Read the model definition and answer for the solid it produces. Units are mm, in the model's axes. Face numbers are marked on the shaded views. Round coordinates to 2 decimals unless told otherwise and drop trailing zeros. Write each loop counter-clockwise with the first axis right and the second up, starting at its lowest first coordinate (ties: lowest second). Pieces come first, ordered by that corner, then holes.
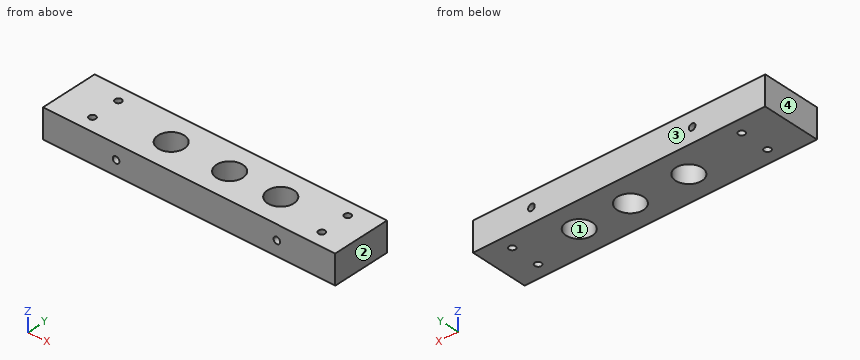
from build123d import *

# Parameters (mm, degrees)
F_200X40X20_START          = -10
SKETCH_1_W                 = 200
SKETCH_1_H                 = 40
F_200X40X20_DEPTH          = 20
CUT_EXTRUDE_321_DEPTH      = 202.246117975
CUT_EXTRUDE_321_DEPTH_BACK = 202.246117975
SKETCH_2_R                 = 9
SKETCH_2_R_2               = 2.25
CUT_EXTRUDE_M4_DEPTH       = 202.246117975
CUT_EXTRUDE_M4_DEPTH_BACK  = 202.246117975
SKETCH_3_R                 = 2.25


with BuildPart() as part:
    # 草图1 → 前臂200x40x20 (new body)
    with BuildSketch(Plane.XY.offset(F_200X40X20_START)):
        with Locations((100, 0)):
            Rectangle(SKETCH_1_W, SKETCH_1_H)
    extrude(amount=F_200X40X20_DEPTH)

    # 草图2 → Cut-Extrude 321 (cut, two sides: drawn at the far end of the back side and taken through both)
    with BuildSketch(Plane.XY.offset(-CUT_EXTRUDE_321_DEPTH_BACK)):
        with Locations((70, 0)):
            Circle(SKETCH_2_R)
        with Locations((110, 0)):
            Circle(SKETCH_2_R)
        with Locations((145, 0)):
            Circle(SKETCH_2_R)
        with Locations((25, -10)):
            Circle(SKETCH_2_R_2)
        with Locations((25, 10)):
            Circle(SKETCH_2_R_2)
        with Locations((182, -10)):
            Circle(SKETCH_2_R_2)
        with Locations((182, 10)):
            Circle(SKETCH_2_R_2)
    extrude(amount=CUT_EXTRUDE_321_DEPTH + CUT_EXTRUDE_321_DEPTH_BACK, mode=Mode.SUBTRACT)

    # 草图3 → 主板托盘竖向M4 (cut, two sides: drawn at the far end of the back side and taken through both)
    with BuildSketch(Plane(origin=(0, 0, 0), x_dir=(1, 0, 0), z_dir=(0, 1, 0)).offset(-CUT_EXTRUDE_M4_DEPTH_BACK)):
        with Locations(Location((50, 0, 0), (0, 0, 270))):
            Circle(SKETCH_3_R)
        with Locations(Location((160, 0, 0), (0, 0, 270))):
            Circle(SKETCH_3_R)
    extrude(amount=CUT_EXTRUDE_M4_DEPTH + CUT_EXTRUDE_M4_DEPTH_BACK, mode=Mode.SUBTRACT)


solid = part.part
Q1. Section C-C (z = 0) is taken. State how many separate pieces and enclosed holes the cut face has, then the cut area to 3 significant figures.
Verdict:
separate pieces: 3
enclosed holes: 7
area: 6,810 mm2
Q2. Section D-D (x = 25) is taken. Determine the outline of the cut face in (y, z), then the cut area to 3 significant figures.
Verdict:
outline: (-20, -10) - (-12.25, -10) - (-12.25, 10) - (-20, 10) - close; (-7.75, -10) - (7.75, -10) - (7.75, 10) - (-7.75, 10) - close; (12.25, -10) - (20, -10) - (20, 10) - (12.25, 10) - close
area: 620 mm2
Q3. Straight lines are drawn through the part: probe 1 along X at (y, z) = (0, -3); probe 2 along X at (y, z) = (-10, 3.5); probe 3 along Y at (x, z) = (182, -4.25). For each, find the intervals that lie inside material, in ascending order.
Verdict:
probe 1: x = 0 to 61, 79 to 101, 119 to 136, 154 to 200
probe 2: x = 0 to 22.75, 27.25 to 179.75, 184.25 to 200
probe 3: y = -20 to -12.25, -7.75 to 7.75, 12.25 to 20
Q4. Determine the mould class of the marked faces 1, 2, 3 and 4 for opening direction X: pulls with the +X half, pulls with the -X half, needs draft (parallel to the pull), parting line crosses it, or undercut.
Verdict:
face 1: undercut
face 2: pulls with the +X half
face 3: needs draft
face 4: pulls with the -X half
Q5. Section A-A (y = 0) is taken. Determine the outline of the cut face in (x, z).
Verdict:
outline: (0, -10) - (61, -10) - (61, 10) - (0, 10) - close; (79, -10) - (101, -10) - (101, 10) - (79, 10) - close; (119, -10) - (136, -10) - (136, 10) - (119, 10) - close; (154, -10) - (200, -10) - (200, 10) - (154, 10) - close; hole circle Ø4.5 at (50, 0); hole circle Ø4.5 at (160, 0)
Q6. Section B-B (x = 50) is taken. Determine the outline of the cut face in (y, z), then the cut area to 3 significant figures.
Verdict:
outline: (-20, -10) - (20, -10) - (20, -2.25) - (-20, -2.25) - close; (-20, 2.25) - (20, 2.25) - (20, 10) - (-20, 10) - close
area: 620 mm2
